Verification items for the finished model (mm, model axes). Round coordinates to 2 decimals unless told otherwise and drop trailing zeros. Loops run counter-clockwise (first coordinate to the right, second up) from the corner with the lowest first, then second, coordinate; pieces in that order, holes last. Notation, with made-up numbers: M 86,22 L 144,22 A27 ccw 144,49 Z; hole C 30,6.25 d7. An arc over 180 degrees is marked long. One line per item, written item: value.
Autodesk Inventor part; units mm, degrees
ref_plane "YZ Plane" through (0, 0, 0) normal (1, 0, 0) x (0, 1, 0)
ref_plane "XZ Plane" through (0, 0, 0) normal (0, 1, 0) x (-1, 0, 0)
ref_plane "XY Plane" through (0, 0, 0) normal (0, 0, 1) x (1, 0, 0)
sketch "Sketch1" plane through (0, 0, 0) normal (0, 1, 0) x (-1, 0, 0)
  line L0 (-4.75, 8.5) -> (4.75, 8.5)
  line L1 (4.75, 8.5) -> (4.75, -8.5)
  line L2 (4.75, -8.5) -> (-4.75, -8.5)
  line L3 (-4.75, -8.5) -> (-4.75, 8.5)
  line L4 (-4.75, 8.5) -> (4.75, -8.5) construction
  line L5 (4.75, 8.5) -> (-4.75, -8.5) construction
  line L6 (0, -8.5) -> (0, -3.5) construction
  circle A0 centre (0, -3.5) radius 2.25
  point P0 (0, 0)
  dimension "d2" = 9.5
  dimension "d3" = 17
  dimension "d4" = 5
  dimension "d5" = 4.5
extrude "Extrusion1" add sketch "Sketch1" along normal blind 5
fillet "Fillet1" radius 5 1 edges at (4.75, 2.5, 8.5)
fillet "Fillet2" radius 5 1 edges at (-4.75, 2.5, 8.5)
fillet "Fillet3" radius 2 2 edges at (-4.75, 2.5, -8.5) (4.75, 2.5, -8.5)
properties part number "Clamp"
(1) Thickness scan on L1, parallel to Z at x = 0, y = 3.2; L2, parallel to Z at x = -2, y = 3.9; L3, parallel to Z at x = -3.5, y = 4.6. Record the ranges inside material, lowest first. Write a range as from..to.
Completed:
L1: z = -8.5..-5.75, -1.25..8.49
L2: z = -8.5..-4.53, -2.47..7.99
L3: z = -8.35..6.83
(2) Sectioned sample at A-A on z = -3.5. Enter the section's corners in (x, y).
Completed:
outline: M -4.75,0 L -2.25,0 L -2.25,5 L -4.75,5 Z; M 2.25,0 L 4.75,0 L 4.75,5 L 2.25,5 Z
(3) Sectioned sample at C-C on x = 0.25. Enter the section's corners in (y, z), and give its area (3 significant figures).
Completed:
outline: M 0,-8.5 L 5,-8.5 L 5,-5.74 L 0,-5.74 Z; M 0,-1.26 L 5,-1.26 L 5,8.47 L 0,8.47 Z
area: 62.5 mm^2
(4) Sectioned sample at D-D on x = 3.75. Enter the section's corners in (y, z), and give its area (3 significant figures).
Completed:
outline: M 0,-8.23 L 5,-8.23 L 5,6.5 L 0,6.5 Z
area: 73.7 mm^2
(5) Mould release check, pull along Z, two halves, no side actions. Record for faces 1 (the face through (0.488, 2.465, -1.304)), 2 (the face through (4.75, 2, -2)), 3 (the face through (-3.42, 2.46, 6.92)): +Z half, -Z half, draft (parallel to the pull), parting line (faces both ways), or undercut.
Completed:
face 1: undercut
face 2: draft
face 3: +Z half
(6) Sectioned sample at B-B on y = 4.2. Enter the section's corners in (x, z).
Completed:
outline: M -4.75,-6.5 A2 ccw -2.75,-8.5 L 2.75,-8.5 A2 ccw 4.75,-6.5 L 4.75,3.5 A5 ccw -0.25,8.5 A5 ccw -4.75,3.53 Z; hole C 0,-3.5 d4.5
